from build123d import *

# Parameters (mm, degrees)
SKETCH_3_R          = 9.5
EXTRUDE_1_DEPTH     = 2
EXTRUDE_START       = -2
EXTRUDE_2_DEPTH     = 2
FILLET_2_R          = 13
SKETCH_5_R          = 1.15
CUT_EXTRUDE_1_DEPTH = 58.948126493
SKETCH_6_R          = 9.5
CUT_EXTRUDE_2_DEPTH = 58.948126493
FILLET_3_R          = 8
FILLET_4_R          = 7
SKETCH_7_R          = 1.08334678
CUT_EXTRUDE_4_DEPTH = 10
CUT_EXTRUDE_5_DEPTH = 10
FILLET_5_R          = 1


with BuildPart() as part:
    # 草图3 → 凸台-拉伸1 (new body)
    with BuildSketch(Plane.XY):
        with BuildLine():
            Line((-11, 0), (-11, -33))
            Line((-11, -33), (35.74, -33))
            ThreePointArc((35.74, -33), (46.48709263, -19.65479212), (31.157424305, -12))
            Line((31.157424305, -12), (9, -12))
            Line((9, -12), (9, -6.32455532))
            ThreePointArc((9, -6.32455532), (3.31662479, 10.488088482), (-11, 0))
        make_face()
        Circle(SKETCH_3_R, mode=Mode.SUBTRACT)
        with Locations((35.74, -22)):
            Circle(SKETCH_3_R, mode=Mode.SUBTRACT)
    extrude(amount=EXTRUDE_1_DEPTH)

    # 草图4 → 凸台-拉伸2 (add)
    with BuildSketch(Plane.XY.offset(2).offset(EXTRUDE_START)):
        with BuildLine():
            Line((35.74, -33), (-12.210859555, -34.674480913))
            Line((-12.210859555, -34.674480913), (-11, 0))
            ThreePointArc((-11, 0), (3.31662479, 10.488088482), (9, -6.32455532))
            Line((9, -6.32455532), (9, -12))
            Line((9, -12), (31.157424305, -12))
            ThreePointArc((31.157424305, -12), (46.48709263, -19.65479212), (35.74, -33))
        make_face()
    extrude(amount=EXTRUDE_2_DEPTH)

    # 圆角2
    fillet_2_edges = [part.edges().sort_by_distance(p)[0] for p in [
        (-12.210859555, -34.674480913, 1),
    ]]
    fillet(fillet_2_edges, radius=FILLET_2_R)

    # 草图5 → 切除-拉伸1 (cut, through all)
    with BuildSketch(Plane.XY.offset(2)):
        with Locations((-8, -22.5)):
            Circle(SKETCH_5_R)
        with Locations((8, -22.5)):
            Circle(SKETCH_5_R)
    extrude(amount=-CUT_EXTRUDE_1_DEPTH, mode=Mode.SUBTRACT)

    # 草图6 → 切除-拉伸2 (cut, through all)
    with BuildSketch(Plane.XY.offset(2)):
        Circle(SKETCH_6_R)
        with Locations((35.642814002, -22)):
            Circle(SKETCH_6_R)
    extrude(amount=-CUT_EXTRUDE_2_DEPTH, mode=Mode.SUBTRACT)

    # 圆角3
    # the kernel refuses this fillet: 8 mm, written as the material it adds along each edge
    with BuildSketch(Plane(origin=(9, -12, 0), x_dir=(0, 1, 0), z_dir=(0, 0, 1))) as fillet_3_piece_1:
        with BuildLine():
            CenterArc((8, -7.654831322), FILLET_3_R, 106.89204914, 73.10795086)
            Line((0, -7.654831322), (-0.16, -7.654831322))
            Line((-0.16, -7.654831322), (-0.16, 0))
            Line((-0.16, 0), (0, 0.16))
            ThreePointArc((0, 0.16), (2.83772234, 0.16), (5.628953573, 0.153096626))
            Line((5.628953573, 0.153096626), (5.67544468, 0))
        make_face()
    extrude(amount=2)

    # 圆角4
    fillet_4_edges = [part.edges().sort_by_distance(p)[0] for p in [
        (9, -6.32455532, 1),
    ]]
    fillet(fillet_4_edges, radius=FILLET_4_R)

    # 草图7 → 切除-拉伸4 (cut)
    with BuildSketch(Plane.XY.offset(2)):
        with Locations((13.142814002, -14)):
            Circle(SKETCH_7_R)
        with Locations((13.142814002, -30)):
            Circle(SKETCH_7_R)
    extrude(amount=-CUT_EXTRUDE_4_DEPTH, mode=Mode.SUBTRACT)

    # 草图8 → 切除-拉伸5 (cut)
    with BuildSketch(Plane.XY.offset(2)):
        with BuildLine():
            Line((16.646480101, -26.883817545), (16.646480101, -14.57255416))
            Line((16.646480101, -14.57255416), (22.737666516, -14.57255416))
            ThreePointArc((22.737666516, -14.57255416), (24.403604511, -15.465914835), (24.581259014, -17.347903565))
            ThreePointArc((24.581259014, -17.347903565), (23.697285572, -20.857918339), (23.900157183, -24.47184361))
            ThreePointArc((23.900157183, -24.47184361), (23.496100815, -26.143986607), (21.943047713, -26.883817545))
            Line((21.943047713, -26.883817545), (16.646480101, -26.883817545))
        make_face()
        with BuildLine():
            Line((-1.844212644, -26.7628803), (8.691309214, -26.7628803))
            ThreePointArc((8.691309214, -26.7628803), (9.751969386, -27.202220128), (10.191309214, -28.2628803))
            Line((10.191309214, -28.2628803), (10.191309214, -30.26653293))
            ThreePointArc((10.191309214, -30.26653293), (9.751969386, -31.327193102), (8.691309214, -31.76653293))
            Line((8.691309214, -31.76653293), (-1.844212644, -31.76653293))
            ThreePointArc((-1.844212644, -31.76653293), (-2.904872816, -31.327193102), (-3.344212644, -30.26653293))
            Line((-3.344212644, -30.26653293), (-3.344212644, -28.2628803))
            ThreePointArc((-3.344212644, -28.2628803), (-2.904872816, -27.202220128), (-1.844212644, -26.7628803))
        make_face()
        with BuildLine():
            Line((-8.796911022, -16.052867786), (-8.796911022, -12.380312846))
            ThreePointArc((-8.796911022, -12.380312846), (-7.815486406, -10.659120182), (-5.834406834, -10.627148368))
            ThreePointArc((-5.834406834, -10.627148368), (0.968228408, -12.084664633), (7.452020697, -9.562634212))
            ThreePointArc((7.452020697, -9.562634212), (7.978826228, -9.507761331), (8.259361329, -9.957022011))
            Line((8.259361329, -9.957022011), (8.259361329, -10.859557769))
            ThreePointArc((8.259361329, -10.859557769), (7.914413338, -11.982412545), (6.99855848, -12.717940822))
            Line((6.99855848, -12.717940822), (-6.057713871, -17.911250839))
            ThreePointArc((-6.057713871, -17.911250839), (-7.919765799, -17.707919794), (-8.796911022, -16.052867786))
        make_face()
    extrude(amount=-CUT_EXTRUDE_5_DEPTH, mode=Mode.SUBTRACT)

    # 圆角5
    fillet_5_edges = [part.edges().sort_by_distance(p)[0] for p in [
        (16.646480101, -26.883817545, 1),
        (16.646480101, -14.57255416, 1),
    ]]
    fillet(fillet_5_edges, radius=FILLET_5_R)


solid = part.part
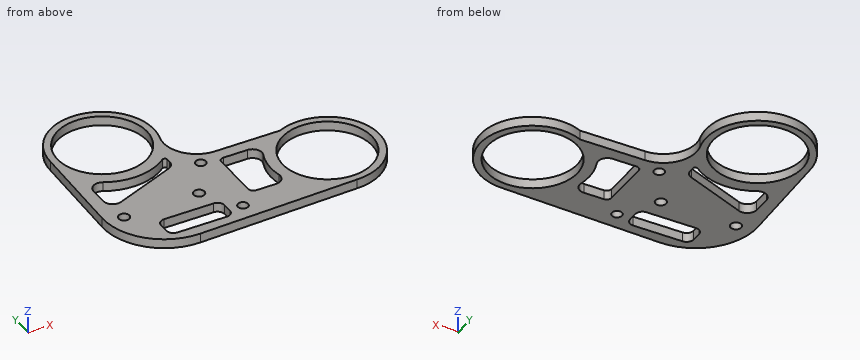
Geometry check sheet. Reference: the model listing, model coordinates, mm. Coordinates: 2 decimals unless noted, no trailing zeros. Order: outer loops, then holes, each group sorted by start corner. A loop starts at its lowest first (then second) coordinate and runs counter-clockwise, first axis right, second up. Notation, with made-up numbers: (84.5, 51) - (111.5, 51) arc R13 cw to (111.5, 56) - close; hole circle Ø7 at (48, 62). An arc over 180 degrees is marked (long way). Answer in a Markdown table with one row per item. Add a question column.
1) Cross-section at A-A, the plane x = 0. Record the cut outline in (y, z).
2) Material ranges on line 1 along Y through (x, z) = (2, 1.9); line 2 along X through (y, z) = (-26, 1.4); line 3 along Y through (x, z) = (8, 1.2), recorded low to high. Write a range as [from, to].
3) Cross-section at D-D, the plane x = -8. Record the cut outline in (y, z), then the cut area to 3 significant figures.
4) Cross-section at C-C, the plane x = 43. Record the cut outline in (y, z).
5) Cross-section at B-B, the plane y = 3. Record the cut outline in (x, z), then the cut area to 3 significant figures.
6) Gauge pin test, flat ends, axial feed: P1, Ø0.6, axis at y = -29.5, z = 1.5, coming from the -X side; P2, Ø1, axis at y = -8, z = 0.5, coming from the +X side; P3, Ø0.6, axis at x = 3, z = 0.5, coming from the +Y side. Record the tip position at first contact, or that the pin passes through.
Check result:
| question | item | result |
|---|---|---|
| 1 | outline | (-34.13, 0) - (-31.77, 0) - (-31.77, 2) - (-34.13, 2) - close; (-26.76, 0) - (-15.5, 0) - (-15.5, 2) - (-26.76, 2) - close; (-12.12, 0) - (-9.5, 0) - (-9.5, 2) - (-12.12, 2) - close; (9.5, 0) - (11, 0) - (11, 2) - (9.5, 2) - close |
| 2 | line 1 | y = [-34.18, -31.77], [-26.76, -14.71], [-11.96, -9.29], [9.29, 10.82] |
| 2 | line 2 | x = [-10.81, 16.65], [23.6, 27.03], [44.26, 45.99] |
| 2 | line 3 | y = [-33.97, -31.77], [-26.76, -23.65], [-21.35, -11.84], [-9.52, -5.12], [5.12, 7.55] |
| 3 | outline | (-30.31, 0) - (-23.65, 0) - (-23.65, 2) - (-30.31, 2) - close; (-21.35, 0) - (-17.65, 0) - (-17.65, 2) - (-21.35, 2) - close; (-10.78, 0) - (-5.12, 0) - (-5.12, 2) - (-10.78, 2) - close; (5.12, 0) - (7.55, 0) - (7.55, 2) - (5.12, 2) - close |
| 3 | area | 36.9 mm² |
| 4 | outline | (-30.26, 0) - (-28.01, 0) - (-28.01, 2) - (-30.26, 2) - close; (-15.99, 0) - (-13.74, 0) - (-13.74, 2) - (-15.99, 2) - close |
| 5 | outline | (-10.58, 0) - (-9.01, 0) - (-9.01, 2) - (-10.58, 2) - close; (9.01, 0) - (10.58, 0) - (10.58, 2) - (9.01, 2) - close |
| 5 | area | 6.28 mm² |
| 6 | P1 | stops at x = -8.98 |
| 6 | P2 | stops at x = 11.23 |
| 6 | P3 | stops at y = 10.66 |
